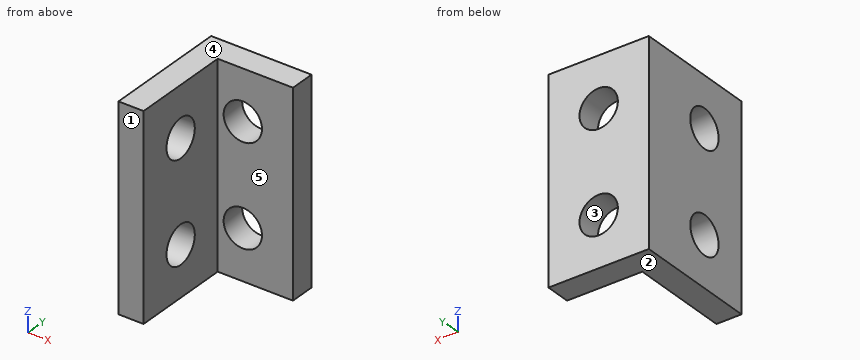
Autodesk Inventor part; units mm, degrees
ref_plane "YZ Plane" through (0, 0, 0) normal (1, 0, 0) x (0, 1, 0)
ref_plane "XZ Plane" through (0, 0, 0) normal (0, 1, 0) x (-1, 0, 0)
ref_plane "XY Plane" through (0, 0, 0) normal (0, 0, 1) x (1, 0, 0)
sketch "Sketch1" plane through (0, 0, 0) normal (0, 0, 1) x (1, 0, 0)
  line L0 (6.35, -7.9375) -> (-6.35, -7.9375)
  line L1 (-6.35, -7.9375) -> (-6.35, 7.9375)
  line L2 (-6.35, 7.9375) -> (6.35, 7.9375)
  line L3 (6.35, 7.9375) -> (6.35, -7.9375)
  line L4 (6.35, -7.9375) -> (-6.35, 7.9375) construction
  line L5 (-6.35, -7.9375) -> (6.35, 7.9375) construction
  line L6 (6.35, -7.9375) -> (-3.175, -7.9375)
  line L7 (-3.175, -7.9375) -> (-3.175, 4.7625)
  line L8 (-3.175, 4.7625) -> (6.35, 4.7625)
  line L9 (6.35, 4.7625) -> (6.35, -7.9375)
  point P0 (0, 0)
  point P1 (-3.175, -7.9375)
  dimension "d0" = 12.7
  dimension "d1" = 15.875
  dimension "d2" = 9.525
  dimension "d3" = 12.7
extrude "Extrusion1" add sketch "Sketch1" along normal blind 25.4 contours L0 L1 L2 L3 L8 L7
sketch "Sketch2" plane through (-3.175, 4.7625, 0) normal (0, -1, 0) x (1, 0, 0)
  circle A0 centre (3.175, 19.05) radius 2.4257
  circle A1 centre (3.175, 6.35) radius 2.4257
  line L0 (0, 25.4) -> (9.525, 25.4)
  line L1 (0, 0) -> (9.525, 0)
  point P0 (3.175, 0)
  point P1 (4.7625, 25.4)
  dimension "d6" = 4.8514
  dimension "d7" = 4.8514
  dimension "d8" = 6.35
  dimension "d9" = 6.35
extrude "Extrusion2" cut sketch "Sketch2" against normal blind 25.4
sketch "Sketch3" plane through (-3.175, -7.9375, 0) normal (1, 0, 0) x (0, 0, -1)
  circle A0 centre (-6.35, 6.35) radius 2.4257
  circle A1 centre (-19.05, 6.35) radius 2.4257
  line L0 (-25.4, 0) -> (-25.4, 12.7)
  line L1 (0, 0) -> (0, 12.7)
  point P0 (0, 7.9375)
  dimension "d12" = 4.8514
  dimension "d13" = 4.8514
  dimension "d14" = 6.35
  dimension "d15" = 6.35
extrude "Extrusion3" cut sketch "Sketch3" against normal blind 25.4
properties part number "Gusset" material "Stainless Steel"
Design review of the part built by this model. Coordinates are the model's own, in mm. Face numbers are marked on the shaded views. A direction names the side the tool comes from. Coordinates: 2 decimals unless noted, no trailing zeros. Write each loop counter-clockwise with the first axis right and the second up, starting at its lowest first coordinate (ties: lowest second). Pieces come first, ordered by that corner, then holes. Notation, with made-up numbers: (36.25, -15) - (95.25, -15) arc R17 ccw to (95.25, 10) - close; hole circle Ø9 at (49, -10.75). An arc over 180 degrees is marked (long way). One line per item, written item: value.
1) For the marked faces 4 and 5, list the 3-axis set-ups (+Z, -Z, +X, -X, +Y, -Y) from which the entire face can be reached by the end or side of a thin tool; tool diameter is ignored.
Answer sheet:
face 4: +Z, +X, -X, +Y, -Y
face 5: +Z, -Z, +X, -Y
2) Add section A-A (x = 0). State the section outline as (y, z) points, plus the area to 3 significant figures.
Answer sheet:
outline: (4.76, 0) - (7.94, 0) - (7.94, 3.92) - (4.76, 3.92) - close; (4.76, 8.78) - (7.94, 8.78) - (7.94, 16.62) - (4.76, 16.62) - close; (4.76, 21.48) - (7.94, 21.48) - (7.94, 25.4) - (4.76, 25.4) - close
area: 49.8 mm2
3) Add section B-B (z = 19.05). Give the number of separate pieces and of enclosed holes in the cut face, plus the area to 3 significant figures.
Answer sheet:
separate pieces: 3
enclosed holes: 0
area: 49.8 mm2
4) Insertion check: pin 1 (5 mm diameter, centred on x = 0, z = 11.5, fed in from -Y); pin 2 (4 mm diameter, centred on y = -1.59, z = 6.35, fed in from +X); pin 3 (4 mm diameter, centred on y = -0.5, z = 19, fed in from +X) (3 decimals). Each pin has a flat end and moves straight along its axis. Give the tip position at first contact, or say it passes through.
Answer sheet:
pin 1: stops at y = 4.76
pin 2: passes through
pin 3: stops at x = -3.175
5) Mouldability with a two-part tool opening along Z and no side actions: class the marked faces 1, 2 and 3 as +Z half, -Z half, draft (parallel to the pull), parting line (faces both ways), or undercut.
Answer sheet:
face 1: draft
face 2: -Z half
face 3: undercut
6) Add section D-D (y = -2). State the section outline as (x, z) points (3 decimals).
Answer sheet:
outline: (-6.35, 0) - (-3.175, 0) - (-3.175, 3.96) - (-6.35, 3.96) - close; (-6.35, 8.74) - (-3.175, 8.74) - (-3.175, 16.66) - (-6.35, 16.66) - close; (-6.35, 21.44) - (-3.175, 21.44) - (-3.175, 25.4) - (-6.35, 25.4) - close
7) To check wall thickness, follow probe 1 along Z at (x, y) = (0, 5.7); probe 2 along X at (y, z) = (0, 23.75) (3 decimals); probe 3 along Y at (x, z) = (-4.95, 6.35). State the ranges of each line that lie inside material, in increasing order.
Answer sheet:
probe 1: z = 0 to 3.92, 8.78 to 16.62, 21.48 to 25.4
probe 2: x = -6.35 to -3.175
probe 3: y = -7.94 to -4.01, 0.84 to 7.94
